Work out the finished part from the listing and answer in its coordinate system (mm). A direction names the side the tool comes from. Round coordinates to 2 decimals unless told otherwise and drop trailing zeros. Order: outer loops, then holes, each group sorted by start corner. A loop starts at its lowest first (then second) coordinate and runs counter-clockwise, first axis right, second up. Notation, with made-up numbers: (14.25, 81.25) - (29.25, 81.25) arc R24 ccw to (29.25, 96.25) - close; hole circle Ø3 at (54.25, -25). An arc over 180 degrees is marked (long way). Answer in a Markdown table with one row per item.
Autodesk Inventor part; units mm, degrees
ref_plane "YZ Plane" through (0, 0, 0) normal (1, 0, 0) x (0, 1, 0)
ref_plane "XZ Plane" through (0, 0, 0) normal (0, 1, 0) x (-1, 0, 0)
ref_plane "XY Plane" through (0, 0, 0) normal (0, 0, 1) x (1, 0, 0)
sketch "Sketch1" plane through (0, 0, 0) normal (0, 1, 0) x (-1, 0, 0)
  circle A0 centre (0, 0) radius 5
  dimension "d0" = 10
sketch "Sketch2" plane through (0, 0, 0) normal (0, 1, 0) x (-1, 0, 0)
  point P0 (0, 0)
extrude "Extrusion1" add sketch "Sketch1" along normal blind 1.5
sketch "Sketch3" plane through (0, 1.5, 0) normal (0, 1, 0) x (1, 0, 0)
  circle A0 centre (0, 0) radius 4.5
  circle A1 centre (0, 0) radius 5
  dimension "d3" = 9
extrude "Extrusion2" add sketch "Sketch3" along normal blind 7
sketch "Sketch4" plane through (0, 1.5, 0) normal (0, 1, 0) x (1, 0, 0)
  line L0 (3, 3) -> (3.5, 3)
  line L1 (3.5, 3) -> (3.5, 2)
  line L2 (3.5, 2) -> (3, 2)
  line L3 (3, 2) -> (3, 3)
  line L4 (3, 3) -> (3.5, 2) construction
  line L5 (3.5, 3) -> (3, 2) construction
  line L6 (-3.5, 3) -> (-3, 3)
  line L7 (-3, 3) -> (-3, 2)
  line L8 (-3, 2) -> (-3.5, 2)
  line L9 (-3.5, 2) -> (-3.5, 3)
  line L10 (-3.5, 3) -> (-3, 2) construction
  line L11 (-3, 3) -> (-3.5, 2) construction
  line L12 (-3.5, -2) -> (-3, -2)
  line L13 (-3, -2) -> (-3, -3)
  line L14 (-3, -3) -> (-3.5, -3)
  line L15 (-3.5, -3) -> (-3.5, -2)
  line L16 (-3.5, -2) -> (-3, -3) construction
  line L17 (-3, -2) -> (-3.5, -3) construction
  line L18 (3, -2) -> (3.5, -2)
  line L19 (3.5, -2) -> (3.5, -3)
  line L20 (3.5, -3) -> (3, -3)
  line L21 (3, -3) -> (3, -2)
  point P0 (0, 0)
  point P1 (3.25, 2.5)
  point P2 (-3.25, 2.5)
  point P3 (-3.25, -2.5)
  dimension "d8" = 0.5
  dimension "d9" = 1
  dimension "d10" = 0.5
  dimension "d11" = 1
  dimension "d12" = 0.5
  dimension "d13" = 1
  dimension "d15" = 6
  dimension "d16" = 7
  dimension "d17" = 0
  dimension "d18" = 0
  dimension "d20" = 0.5
  dimension "d21" = 1
  dimension "d22" = 7
  dimension "d23" = 0
  dimension "d24" = 3.5
  dimension "d26" = 3
extrude "Extrusion3" cut sketch "Sketch4" against normal blind 7
properties part number "button_bottom"
1) The mould has two halves that part along Z. Classify faces 1 (the face through (0, 1.5, 0)), 2 (the face through (0, 4, 5)), 3 (the face through (0, 0, 0)): released by +Z, released by -Z, zero draft, split by the parting line, or undercut.
Filled in:
| item | result |
|---|---|
| face 1 | undercut |
| face 2 | split by the parting line |
| face 3 | zero draft |
2) Find the intervals of material crossed by probe 1 along Z at (x, y) = (0, 3); probe 2 along X at (y, z) = (1, -2.5), in increasing order. Write a range as from..to.
Filled in:
| item | result |
|---|---|
| probe 1 | z = -5..-4.5, 4.5..5 |
| probe 2 | x = -4.33..-3.5, -3..3, 3.5..4.33 |
3) Find section A-A, the plane y = 2. Give the vertices of the cut face in (x, z), then the cut area to 3 significant figures.
Filled in:
| item | result |
|---|---|
| outline | circle Ø10 at (0, 0); hole circle Ø9 at (0, 0) |
| area | 14.9 mm^2 |
4) Each of these flat-tipped pins is pushed along its axis until it touches: pin 1 (0.5 mm diameter, centred on y = 1, z = -2.5, fed in from -X); pin 2 (1.1 mm diameter, centred on y = 0.5, z = -2.5, fed in from -X); pin 3 (1.1 mm diameter, centred on y = 0.5, z = 2.5, fed in from +X). Where does it stop, or does it pass through?
Filled in:
| item | result |
|---|---|
| pin 1 | stops at x = -4.47 |
| pin 2 | stops at x = -4.6 |
| pin 3 | stops at x = 4.6 |
5) Which of the six approach directions +Z, -Z, +X, -X, +Y, -Y give full straight-line access (tool end or side, diameter ignored) to faces 4 (the face through (-3.5, 0.8, 2.5)), 5 (the face through (3, 0.8, 2.5)), 6 (the face through (-0.59, 4.95, 4.46))?
Filled in:
| item | result |
|---|---|
| face 4 | -Y |
| face 5 | +Y, -Y |
| face 6 | +Y |
6) Find section B-B, the plane z = -1. Give the vertices of the cut face in (x, y).
Filled in:
| item | result |
|---|---|
| outline | (-4.9, 0) - (4.9, 0) - (4.9, 8.5) - (4.39, 8.5) - (4.39, 1.5) - (-4.39, 1.5) - (-4.39, 8.5) - (-4.9, 8.5) - close |
